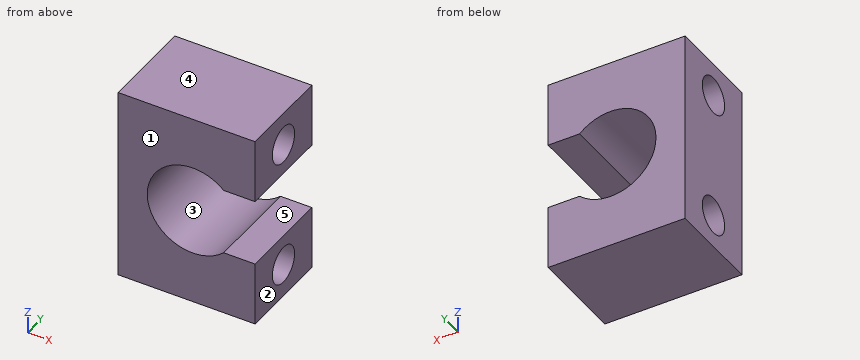
from build123d import *

# Parameters (mm, degrees)
SKETCH1_W           = 20.32
SKETCH1_H           = 28.93
BOSS_EXTRUDE1_DEPTH = 14.02
CUT_EXTRUDE1_DEPTH  = 15.02
SKETCH3_R           = 2.75
CUT_EXTRUDE2_DEPTH  = 21.32


with BuildPart() as part:
    # Sketch1 → Boss-Extrude1 (new body)
    with BuildSketch(Plane(origin=(0, 0, 0), x_dir=(1, 0, 0), z_dir=(0, 1, 0))):
        Rectangle(SKETCH1_W, SKETCH1_H)
    extrude(amount=BOSS_EXTRUDE1_DEPTH)

    # Sketch2 → Cut-Extrude1 (cut, through all)
    with BuildSketch(Plane(origin=(0, 14.02, 0), x_dir=(1, 0, 0), z_dir=(0, 1, 0))):
        with BuildLine():
            Line((10.16, -4.95), (5.499117562, -4.95))
            ThreePointArc((5.499117562, -4.95), (-5.84, 0), (5.499117562, 4.95))
            Line((5.499117562, 4.95), (10.16, 4.95))
            Line((10.16, 4.95), (10.16, -4.95))
        make_face()
    extrude(amount=-CUT_EXTRUDE1_DEPTH, mode=Mode.SUBTRACT)

    # Sketch3 → Cut-Extrude2 (cut, through all)
    with BuildSketch(Plane.ZY.offset(10.16)):
        with Locations((9.525, 7.01)):
            Circle(SKETCH3_R)
        with Locations((-9.525, 7.01)):
            Circle(SKETCH3_R)
    extrude(amount=-CUT_EXTRUDE2_DEPTH, mode=Mode.SUBTRACT)


solid = part.part
The listing builds one solid part. Answer for the finished solid, in the listing's coordinates (mm). Face numbers are marked on the shaded views. A direction names the side the tool comes from. Give positions to 0.01 mm unless a question says otherwise; leave off trailing zeros. Order: outer loops, then holes, each group sorted by start corner. A loop starts at its lowest first (then second) coordinate and runs counter-clockwise, first axis right, second up. Notation, with made-up numbers: (18.5, 16.25) - (49.5, 16.25) arc R15 ccw to (49.5, 32.25) - close; hole circle Ø8 at (88.5, 75.5). An arc over 180 degrees is marked (long way). Use one line per item in the form item = value.
1) Find section D-D on x = -7.25. Determine the outline of the cut face in (y, z) (3 decimals), and give its area (3 significant figures).
Verdict:
outline = (0, -14.465) - (14.02, -14.465) - (14.02, 14.465) - (0, 14.465) - close; hole circle Ø5.5 at (7.01, -9.525); hole circle Ø5.5 at (7.01, 9.525)
area = 358 mm^2
2) Find section B-B on y = 7.01. Determine the outline of the cut face in (x, z) (3 decimals).
Verdict:
outline = (-10.16, -14.465) - (10.16, -14.465) - (10.16, -12.275) - (-10.16, -12.275) - close; (-10.16, -6.775) - (10.16, -6.775) - (10.16, -4.95) - (5.499, -4.95) arc R6.75 cw (long way) to (5.499, 4.95) - (10.16, 4.95) - (10.16, 6.775) - (-10.16, 6.775) - close; (-10.16, 12.275) - (10.16, 12.275) - (10.16, 14.465) - (-10.16, 14.465) - close
3) The mould has two halves that part along X. Classify the marked faces 1, 2 and 3: released by +X, released by -X, zero draft, split by the parting line, or undercut.
Verdict:
face_1 = zero draft
face_2 = released by +X
face_3 = undercut
4) Consider probe 1 along Y at (x, z) = (-4.75, -9.5); probe 2 along Z at (x, y) = (3.5, 7.75) (3 decimals); probe 3 along Z at (x, y) = (-5, 5.75) (3 decimals). Determine where each line is inside the solid, lowest interval first. Write a range as [from, to].
Verdict:
probe_1 = [0, 4.26], [9.76, 14.02]
probe_2 = [-14.465, -12.174], [-6.876, -6.233], [6.233, 6.876], [12.174, 14.465]
probe_3 = [-14.465, -11.969], [-7.081, -3.261], [3.261, 7.081], [11.969, 14.465]
5) For the marked faces 4 and 5, determine the directions among +Z, -Z, +X, -X, +Y, -Y from which every point of the face is accessible in a straight line to the end or side of a thin tool.
Verdict:
face_4 = +Z, +X, -X, +Y, -Y
face_5 = +X, +Y, -Y
6) This flat-tipped pin is pushed along its axis until it touches: pin 1 (4.5 mm diameter, centred on y = 7.01, z = -9.525, fed in from +X). Where does it stop, or does it pass through?
Verdict:
pin_1 = through
7) Find section C-C on z = -6. Determine the outline of the cut face in (x, y).
Verdict:
outline = (-10.16, 0) - (-2.18, 0) - (-2.18, 14.02) - (-10.16, 14.02) - close; (4, 0) - (10.16, 0) - (10.16, 14.02) - (4, 14.02) - close
8) Find section A-A on x = 8.75. Determine the outline of the cut face in (y, z) (3 decimals), and give its area (3 significant figures).
Verdict:
outline = (0, -14.465) - (14.02, -14.465) - (14.02, -4.95) - (0, -4.95) - close; (0, 4.95) - (14.02, 4.95) - (14.02, 14.465) - (0, 14.465) - close; hole circle Ø5.5 at (7.01, -9.525); hole circle Ø5.5 at (7.01, 9.525)
area = 219 mm^2
